Here's how the part is built. I have some questions about the finished solid (model axes, mm). A direction names the side the tool comes from. Give positions to 0.01 mm unless a question says otherwise; leave off trailing zeros. Order: outer loops, then holes, each group sorted by start corner. A loop starts at its lowest first (then second) coordinate and runs counter-clockwise, first axis right, second up. Notation, with made-up numbers: (35, 76) -> (73, 76) arc R8 ccw to (73, 86) -> close; hole circle Ø7 at (-19.75, 70.25). An arc over 180 degrees is marked (long way). Write each question's results on one line, items separated by ' | '. Start each with the question number.
Q1. Imagine slicing it at C-C, the plane z = 5.75. Please give me the cut outline in (x, y), then the cut area to 3 significant figures.
Q2. Thinking about a two-plate mould opening in Z: for faces 1 (the face through (-2.05, -9.25, 5.75)), 2 (the face through (-0.878, -3.954, 0.986)), 3 (the face through (0, 0, 0)), which applies, pulls with the +Z half, pulls with the -Z half, needs draft (parallel to the pull), parting line crosses it, or undercut?
Q3. I need wall thicknesses on line 1 along Z through (x, y) = (5, -4.25); line 2 along Y through (x, z) = (-3.25, 1.5); line 3 along X through (y, z) = (-3, 3.5). Which ranges of each line are inside material? Lowest first, please. Write a range as [from, to].
Q4. Imagine slicing it at A-A, the plane y = 0. Please give me the cut outline in (x, z).
Q5. I'm going to push flat-ended pins straight in: pin 1 (1 mm diameter, centred on x = -4, z = 5.5, fed in from -Y); pin 2 (3 mm diameter, centred on x = 6.5, z = 2, fed in from -Y); pin 3 (2 mm diameter, centred on x = -6, z = 1.5, fed in from +Y). Where does each tip first touch, or does it pass through?
Q6. For faces 4 (the face through (4.3, 0.1, 2)), 5 (the face through (0, 0, 8)), which set-ups out of +Z, -Z, +X, -X, +Y, -Y let a thin tool reach every point of the face, with its end or its side?
```python
from build123d import *

# Parameters (mm, degrees)
ESQUISSE1_R        = 4.05
BOSS_EXTRU_1_DEPTH = 2
ESQUISSE2_R        = 10
BOSS_EXTRU_2_DEPTH = 6
BOSS_EXTRU_2_TAPER = 8
CONG_1_R           = 1


with BuildPart() as part:
    # Esquisse1 → Boss.-Extru.1 (new body)
    with BuildSketch(Plane.XY):
        Circle(ESQUISSE1_R)
    extrude(amount=BOSS_EXTRU_1_DEPTH)

    # Esquisse2 → Boss.-Extru.2 (add)
    with BuildSketch(Plane.XY.offset(2)):
        Circle(ESQUISSE2_R)
    extrude(amount=BOSS_EXTRU_2_DEPTH, taper=BOSS_EXTRU_2_TAPER)

    # Congé1
    cong_1_edges = [part.edges().sort_by_distance(p)[0] for p in [
        (-9.156754992, 0, 8),
    ]]
    fillet(cong_1_edges, radius=CONG_1_R)


solid = part.part
```
Geometry check:
1) outline: circle Ø18.95 at (0, 0) | area: 282 mm²
2) face 1: pulls with the +Z half | face 2: needs draft | face 3: pulls with the -Z half
3) line 1: [2, 8] | line 2: [-2.42, 2.42] | line 3: [-9.32, 9.32]
4) outline: (-10, 2) -> (-4.05, 2) -> (-4.05, 0) -> (4.05, 0) -> (4.05, 2) -> (10, 2) -> (9.28, 7.14) arc R1 ccw to (8.29, 8) -> (-8.29, 8) arc R1 ccw to (-9.28, 7.14) -> close
5) pin 1: y = -8.85 | pin 2: y = -8.66 | pin 3: y = 8.58
6) face 4: -Z | face 5: +Z, +X, -X, +Y, -Y
